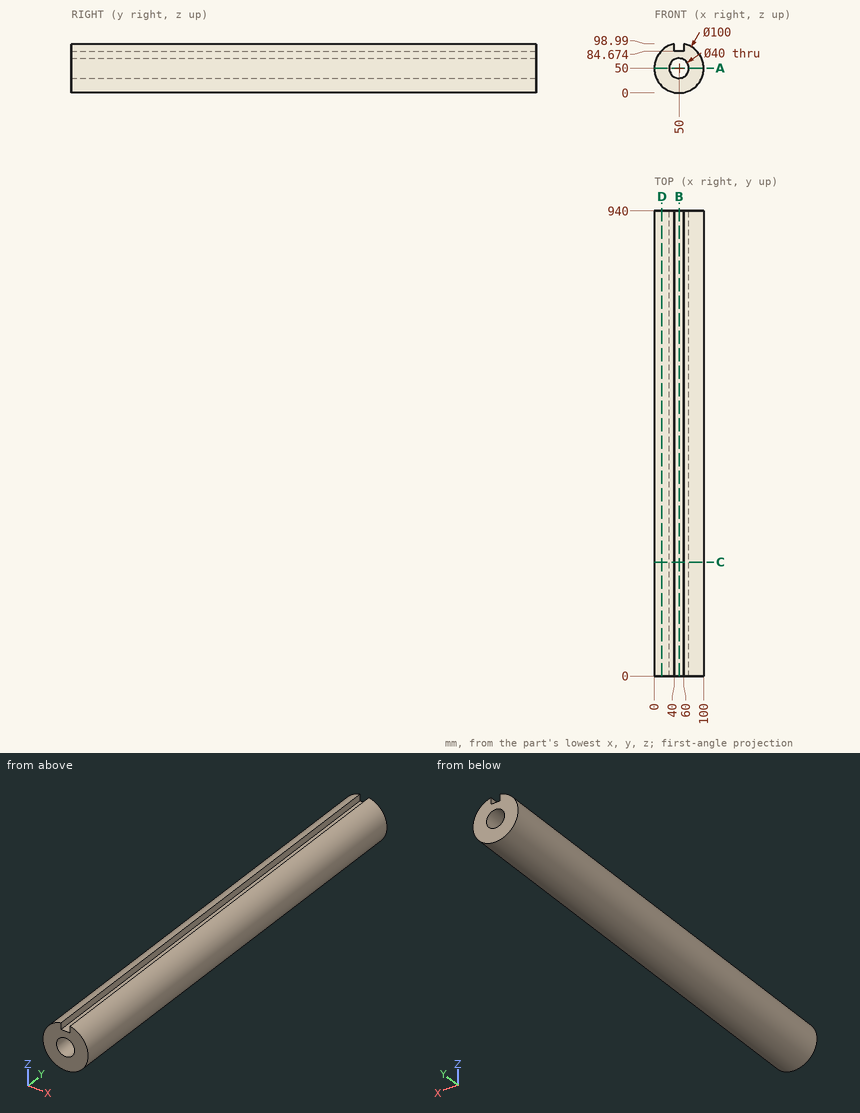
For this review, use the dimensioned drawing (mm, ordinates from the lowest corner) and the shaded views. Round coordinates to 2 decimals unless told otherwise and drop trailing zeros. Order: outer loops, then holes, each group sorted by start corner. A loop starts at its lowest first (then second) coordinate and runs counter-clockwise, first axis right, second up. Notation, with made-up numbers: M 12,35 L 62,35 A20 cw 62,43 Z; hole C -1,2.25 d5. An arc over 180 degrees is marked long. Use a Markdown table: item, result. Add a question column.
Item 1: Add section B-B, the plane x = 50. Give the boundary of the cut face in (y, z), then the cut area to 3 significant figures.
Item 2: Add section A-A, the plane z = 50. Give the boundary of the cut face in (x, y).
Item 3: Add section D-D, the plane x = 15.5. Give the boundary of the cut face in (y, z), then the cut area to 3 significant figures.
Item 4: Insertion check: pin 1 (8 mm diameter, centred on y = 117.5, z = 15, fed in from -X); pin 2 (11.5 mm diameter, centred on y = 241, z = 95.5, fed in from -X); pin 3 (10 mm diameter, centred on y = 179, z = 30.5, fed in from +X). Each pin has a flat end and moves straight along its axis. Give the tip position at first contact, or say it passes through.
Item 5: Add section C-C, the plane y = 230. Give the boundary of the cut face in (x, z), then the cut area to 3 significant figures.
Item 6: To check wall thickness, follow line 1 along Z through (x, y) = (50, 593); line 2 along Z through (x, y) = (34.5, 304); line 3 along X through (y, z) = (373.5, 85). State the ranges of each line that lie inside material, in increasing order.
Geometry results:
| question | item | result |
|---|---|---|
| 1 | outline | M 0,0 L 940,0 L 940,30 L 0,30 Z; M 0,70 L 940,70 L 940,84.67 L 0,84.67 Z |
| 1 | area | 42,000 mm² |
| 2 | outline | M 0,0 L 30,0 L 30,940 L 0,940 Z; M 70,0 L 100,0 L 100,940 L 70,940 Z |
| 3 | outline | M 0,13.81 L 940,13.81 L 940,86.19 L 0,86.19 Z |
| 3 | area | 68,000 mm² |
| 4 | pin 1 | stops at x = 10.77 |
| 4 | pin 2 | stops at x = 19.67 |
| 4 | pin 3 | stops at x = 97.85 |
| 5 | outline | M 40,84.67 L 40,98.99 A50 ccw long 60,98.99 L 60,84.67 Z; hole C 50,50 d40 |
| 5 | area | 6,300 mm² |
| 6 | line 1 | z = 0 to 30, 70 to 84.67 |
| 6 | line 2 | z = 2.46 to 37.36, 62.64 to 97.54 |
| 6 | line 3 | x = 14.29 to 40, 60 to 85.71 |
